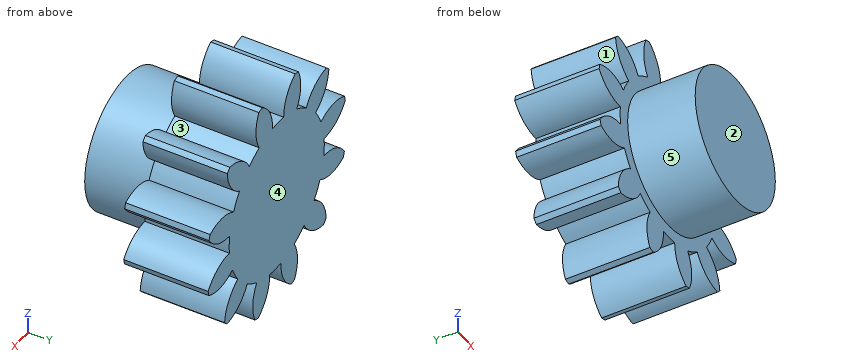
```python
from build123d import *

# Parameters (mm, degrees)
SKETCH1_R           = 4
BOSS_EXTRUDE1_DEPTH = 5
BOSS_EXTRUDE2_START = -9
SKETCH2_R           = 4
BOSS_EXTRUDE2_DEPTH = 9


with BuildPart() as part:
    # Sketch1 → Boss-Extrude1 (new body)
    with BuildSketch(Plane.XZ.offset(5)):
        with BuildLine():
            ThreePointArc((0.852350502, 5.046340911), (-0.292914214, 4.63874602), (-1.091544478, 3.722255668))
            ThreePointArc((-1.091544478, 3.722255668), (-1.570358996, 4.018783876), (-2.080910718, 4.256542705))
            ThreePointArc((-2.080910718, 4.256542705), (-1.75253572, 5.426984811), (-2.039802025, 6.60818883))
            ThreePointArc((-2.039802025, 6.60818883), (-2.208224588, 6.650434309), (-2.377643182, 6.68848927))
            ThreePointArc((-2.377643182, 6.68848927), (-3.165674074, 5.762869382), (-3.399062995, 4.569850323))
            ThreePointArc((-3.399062995, 4.569850323), (-3.961992636, 4.587244025), (-4.523022811, 4.537873349))
            ThreePointArc((-4.523022811, 4.537873349), (-4.823862774, 5.715693447), (-5.663244701, 6.595012981))
            ThreePointArc((-5.663244701, 6.595012981), (-5.830225658, 6.547387358), (-5.995973945, 6.495634624))
            ThreePointArc((-5.995973945, 6.495634624), (-6.215618773, 5.300008841), (-5.821229978, 4.150129568))
            ThreePointArc((-5.821229978, 4.150129568), (-6.317438198, 3.883728135), (-6.778619245, 3.560456788))
            ThreePointArc((-6.778619245, 3.560456788), (-7.628064343, 4.430058932), (-8.794650183, 4.771881024))
            ThreePointArc((-8.794650183, 4.771881024), (-8.915447123, 4.647145545), (-9.033112983, 4.51945222))
            ThreePointArc((-9.033112983, 4.51945222), (-8.625518092, 3.374187504), (-7.709027739, 2.57555724))
            ThreePointArc((-7.709027739, 2.57555724), (-8.005555948, 2.096742722), (-8.243314776, 1.586191))
            ThreePointArc((-8.243314776, 1.586191), (-9.413756883, 1.914565998), (-10.594960902, 1.627299693))
            ThreePointArc((-10.594960902, 1.627299693), (-10.63720638, 1.45887713), (-10.675261342, 1.289458536))
            ThreePointArc((-10.675261342, 1.289458536), (-9.749641454, 0.501427644), (-8.556622395, 0.268038723))
            ThreePointArc((-8.556622395, 0.268038723), (-8.574016096, -0.294890918), (-8.524645421, -0.855921093))
            ThreePointArc((-8.524645421, -0.855921093), (-9.702465518, -1.156761056), (-10.581785053, -1.996142983))
            ThreePointArc((-10.581785053, -1.996142983), (-10.53415943, -2.16312394), (-10.482406696, -2.328872227))
            ThreePointArc((-10.482406696, -2.328872227), (-9.286780912, -2.548517055), (-8.136901639, -2.15412826))
            ThreePointArc((-8.136901639, -2.15412826), (-7.870500207, -2.65033648), (-7.54722886, -3.111517527))
            ThreePointArc((-7.54722886, -3.111517527), (-8.416831004, -3.960962625), (-8.758653095, -5.127548465))
            ThreePointArc((-8.758653095, -5.127548465), (-8.633917617, -5.248345404), (-8.506224291, -5.366011265))
            ThreePointArc((-8.506224291, -5.366011265), (-7.360959576, -4.958416374), (-6.562329312, -4.041926021))
            ThreePointArc((-6.562329312, -4.041926021), (-6.083514793, -4.33845423), (-5.572963071, -4.576213058))
            ThreePointArc((-5.572963071, -4.576213058), (-5.90133807, -5.746655165), (-5.614071764, -6.927859184))
            ThreePointArc((-5.614071764, -6.927859184), (-5.445649202, -6.970104662), (-5.276230608, -7.008159624))
            ThreePointArc((-5.276230608, -7.008159624), (-4.488199715, -6.082539736), (-4.254810795, -4.889520676))
            ThreePointArc((-4.254810795, -4.889520676), (-3.691881154, -4.906914378), (-3.130850979, -4.857543703))
            ThreePointArc((-3.130850979, -4.857543703), (-2.830011016, -6.0353638), (-1.990629088, -6.914683335))
            ThreePointArc((-1.990629088, -6.914683335), (-1.823648131, -6.867057711), (-1.657899844, -6.815304978))
            ThreePointArc((-1.657899844, -6.815304978), (-1.438255016, -5.619679194), (-1.832643812, -4.469799921))
            ThreePointArc((-1.832643812, -4.469799921), (-1.336435592, -4.203398489), (-0.875254545, -3.880127142))
            ThreePointArc((-0.875254545, -3.880127142), (-0.025809446, -4.749729286), (1.140776394, -5.091551377))
            ThreePointArc((1.140776394, -5.091551377), (1.261573333, -4.966815899), (1.379239193, -4.839122573))
            ThreePointArc((1.379239193, -4.839122573), (0.971644302, -3.693857858), (0.05515395, -2.895227594))
            ThreePointArc((0.05515395, -2.895227594), (0.351682158, -2.416413075), (0.589440987, -1.905861353))
            ThreePointArc((0.589440987, -1.905861353), (1.759883093, -2.234236352), (2.941087112, -1.946970046))
            ThreePointArc((2.941087112, -1.946970046), (2.983332591, -1.778547484), (3.021387552, -1.60912889))
            ThreePointArc((3.021387552, -1.60912889), (2.095767664, -0.821097997), (0.902748605, -0.587709077))
            ThreePointArc((0.902748605, -0.587709077), (0.920142307, -0.024779436), (0.870771631, 0.536250739))
            ThreePointArc((0.870771631, 0.536250739), (2.048591729, 0.837090702), (2.927911263, 1.67647263))
            ThreePointArc((2.927911263, 1.67647263), (2.88028564, 1.843453587), (2.828532906, 2.009201874))
            ThreePointArc((2.828532906, 2.009201874), (1.632907123, 2.228846702), (0.48302785, 1.834457906))
            ThreePointArc((0.48302785, 1.834457906), (0.216626417, 2.330666127), (-0.10664493, 2.791847173))
            ThreePointArc((-0.10664493, 2.791847173), (0.762957214, 3.641292272), (1.104779306, 4.807878112))
            ThreePointArc((1.104779306, 4.807878112), (0.980043827, 4.928675051), (0.852350502, 5.046340911))
        make_face()
        with Locations(Location((-3.826936895, -0.159835177, 0), (0, 0, 180))):
            Circle(SKETCH1_R, mode=Mode.SUBTRACT)
    extrude(amount=-BOSS_EXTRUDE1_DEPTH)

    # Sketch2 → Boss-Extrude2 (add)
    with BuildSketch(Plane(origin=(0, 0, 0), x_dir=(1, 0, 0), z_dir=(0, 1, 0)).offset(BOSS_EXTRUDE2_START)):
        with Locations(Location((-3.826936895, 0.159835177, 0), (0, 0, 180))):
            Circle(SKETCH2_R)
    extrude(amount=BOSS_EXTRUDE2_DEPTH)


solid = part.part
```
Source: CAD feature listing. Evaluate the final solid. Frame: model axes, mm. Face numbers are marked on the shaded views. A direction names the side the tool comes from. Give positions to 0.01 mm unless a question says otherwise; leave off trailing zeros. Loops run counter-clockwise (first coordinate to the right, second up) from the corner with the lowest first, then second, coordinate; pieces in that order, holes last. Notation, with made-up numbers: (-19, -14) -> (0, -14) arc R23 ccw to (0, 8) -> close; hole circle Ø3 at (-27.75, 16). An arc over 180 degrees is marked (long way). Put each result on its own line as item: value. Start each with the question number.
1) Cut plane C-C (z = 1). Return loops of the section in (x, y), then the cut area to 3 significant figures.
2) Cut plane A-A (x = 2.25). Return loops of the section in (y, z), then the cut area to 3 significant figures.
3) Contact query for flat-ended pins moving along their axis: P1, Ø2, axis at y = -3.5, z = -4, coming from the -X side; P2, Ø1.5, axis at x = -1.5, y = -4, coming from the +Z side. Output: stop coordinate, or through.
4) Material intervals for probe 1 along Y at (x, z) = (-4.25, -4.25); probe 2 along Z at (x, y) = (2.25, -3); probe 3 along X at (y, z) = (-4.25, -4), sorted ascending.
5) Reachability of the marked faces 1 and 2 from +Z, -Z, +X, -X, +Y, -Y: full face, straight path, thin tool, end or side. Return the list, or none.
6) Cut plane D-D (y = -8). Return loops of the section in (x, z).
7) Cut plane B-B (x = -2.75). Return loops of the section in (y, z), then the cut area to 3 significant figures.
8) Draft query along X for the marked faces 3, 4 and 5. Return one class per face: released by +X, released by -X, zero draft, split by the parting line, or undercut.
Results are:
1. outline: (-10.44, -5) -> (-7.66, -5) -> (-7.66, -9) -> (0, -9) -> (0, -5) -> (2.3, -5) -> (2.3, 0) -> (-10.44, 0) -> close
1. area: 94.3 mm2
2. outline: (-5, -2.19) -> (0, -2.19) -> (0, -0.9) -> (-5, -0.9) -> close; (-5, 0.96) -> (0, 0.96) -> (0, 2.2) -> (-5, 2.2) -> close
2. area: 12.6 mm2
3. P1: stops at x = -8.75
3. P2: stops at z = 6.66
4. probe 1: y = -5 to 0
4. probe 2: z = -2.19 to -0.9, 0.96 to 2.2
4. probe 3: x = -8.44 to -1.03, -0.8 to 1.15
5. face 1: -X, +Y, -Y
5. face 2: +Z, -Z, +X, -X, -Y
6. outline: circle Ø8 at (-3.83, -0.16)
7. outline: (-9, -4.01) -> (-5, -4.01) -> (-5, -6.17) -> (0, -6.17) -> (0, 6.37) -> (-5, 6.37) -> (-5, 3.69) -> (-9, 3.69) -> close
7. area: 93.5 mm2
8. face 3: undercut
8. face 4: zero draft
8. face 5: split by the parting line
